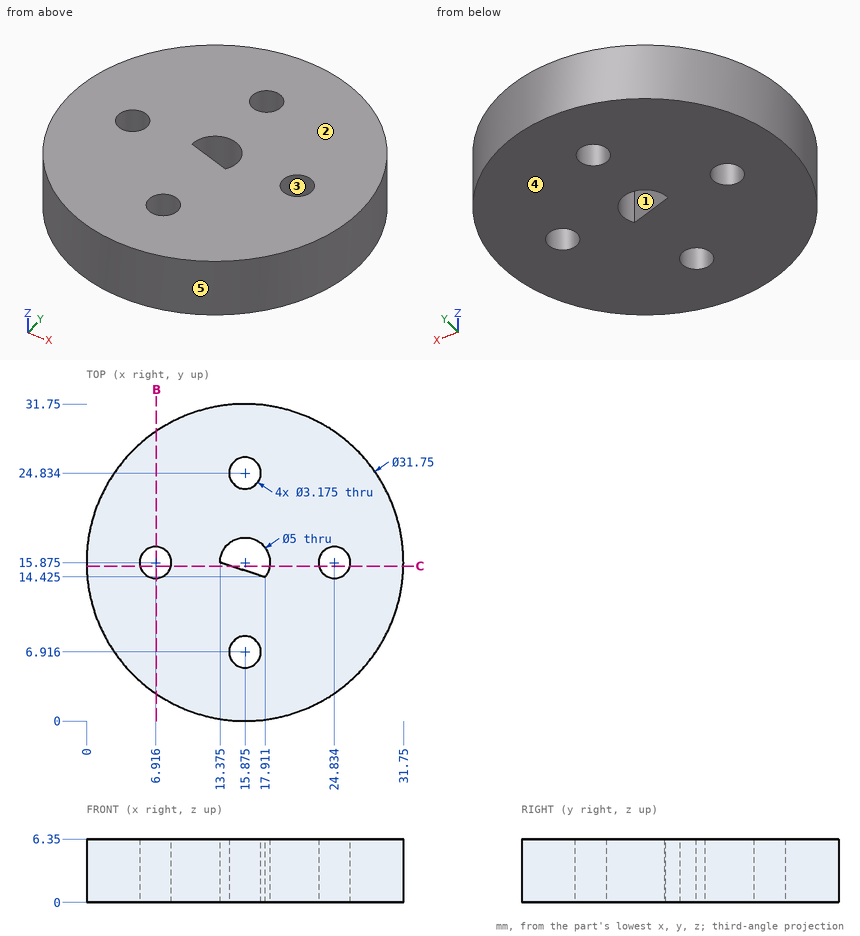
The figure shows three views and two pictorial views of one solid part (mm, origin at its lowest corner). Answer the questions. A direction names the side the tool comes from. Round coordinates to 2 decimals unless told otherwise and drop trailing zeros. Write each loop counter-clockwise with the first axis right and the second up, starting at its lowest first coordinate (ties: lowest second). Pieces come first, ordered by that corner, then holes. Notation, with made-up numbers: M 55.25,37 L 111.25,37 A25 cw 111.25,72 Z; hole C 70,-28 d4. An arc over 180 degrees is marked long. Use a Markdown table: item, result.
1) A tool of negligible diameter and unlimited length cuts with its end or side. For the marked faces 1 and 2, from which of +Z, -Z, +X, -X, +Y, -Y can it reach the whole face along a straight path? Write none if from no direction.
Answers follow:
| item | result |
|---|---|
| face 1 | +Z, -Z |
| face 2 | +Z, +X, -X, +Y, -Y |
2) Flat-ended cylindrical pins translate along their axes: pin 1 (2 mm diameter, centred on y = 13, z = 4.5, fed in from -X); pin 2 (1.5 mm diameter, centred on x = 25, z = 4, fed in from -Y). Find the tip coordinate at first contact, or state that the pin passes through.
Answers follow:
| item | result |
|---|---|
| pin 1 | stops at x = 0.11 |
| pin 2 | stops at y = 2.39 |
3) For a pull along Y with two mould halves and no side action, classify the marked faces 3, 4 and 5 as pulls with the +Y half, pulls with the -Y half, needs draft (parallel to the pull), parting line crosses it, or undercut.
Answers follow:
| item | result |
|---|---|
| face 3 | undercut |
| face 4 | needs draft |
| face 5 | parting line crosses it |
4) The part is cut by section C-C (y = 15.5). Give the number of separate pieces and of enclosed holes in the cut face, plus the area to 3 significant figures.
Answers follow:
| item | result |
|---|---|
| separate pieces | 4 |
| enclosed holes | 0 |
| area | 138 mm2 |
5) Straight lines are drawn through the part: line 1 along X through (y, z) = (25, 4.5) (1 decimal); line 2 along Y through (x, z) = (26, 2.75); line 3 along Y through (x, z) = (18, 4) (1 decimal). For each, find the intervals that lie inside material, in ascending order. Write a range as [from, to].
Answers follow:
| item | result |
|---|---|
| line 1 | x = [2.9, 14.3], [17.5, 28.9] |
| line 2 | y = [3.65, 14.8], [16.95, 28.1] |
| line 3 | y = [0.1, 14.6], [17.2, 31.6] |
6) The part is cut by section B-B (x = 7). Write down the section's boundary in (y, z).
Answers follow:
| item | result |
|---|---|
| outline | M 2.71,0 L 14.29,0 L 14.29,6.35 L 2.71,6.35 Z; M 17.46,0 L 29.04,0 L 29.04,6.35 L 17.46,6.35 Z |
